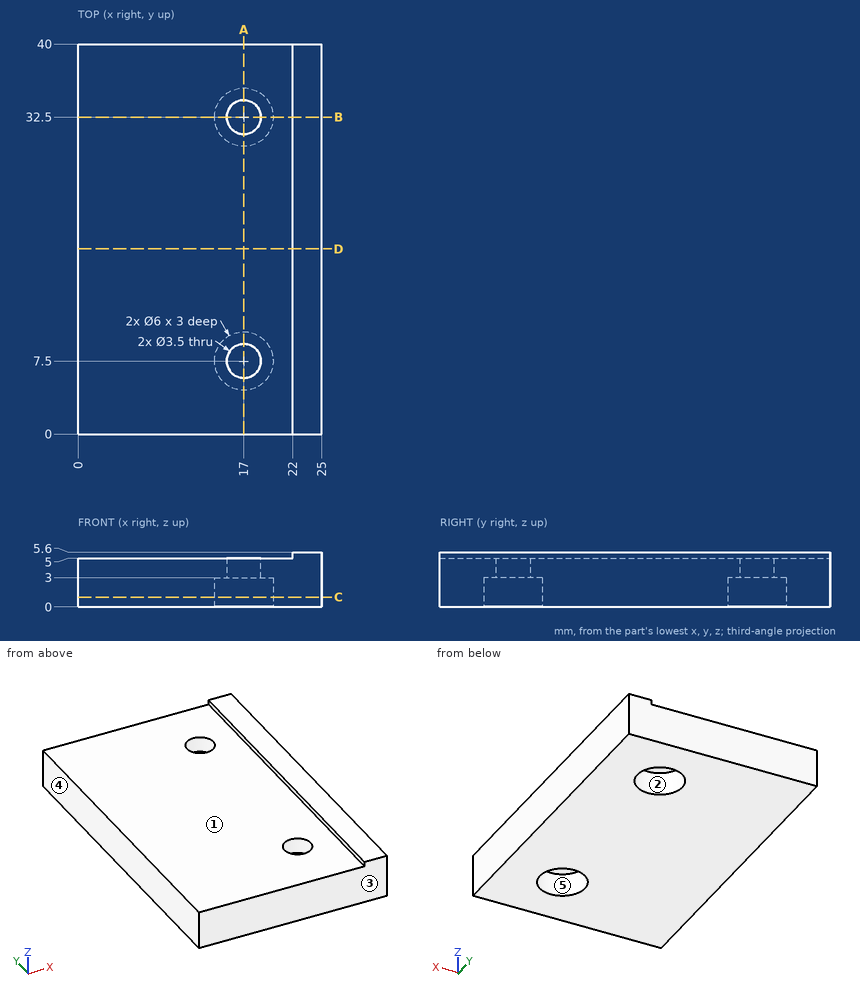
The drawing under review shows one solid part. Ordinate dimensions are in mm from its lowest x, y, z. A direction names the side the tool comes from. Round coordinates to 2 decimals unless told otherwise and drop trailing zeros. Order: outer loops, then holes, each group sorted by start corner. A loop starts at its lowest first (then second) coordinate and runs counter-clockwise, first axis right, second up. Notation, with made-up numbers: (6.25, 3.5) -> (45.25, 3.5) arc R28 cw to (45.25, 32.5) -> close; hole circle Ø3 at (-25.5, -10.5). An arc over 180 degrees is marked (long way). Return JSON: item names as keys, results as strings.
1. The part is to be moulded in two halves that separate along Y. For the marked faces 1, 2 and 3, say which applies: +Y half, -Y half, draft (parallel to the pull), parting line (faces both ways), or undercut.
Answer block:
{"face 1": "draft", "face 2": "undercut", "face 3": "-Y half"}
2. For L1, parallel to Y at x = 17, z = 3.8; L2, parallel to Y at x = 17, z = 0.7; L3, parallel to Z at x = 6.25, y = 6, list the stretches that pass through material, from the lowest coordinate up. Write a range as [from, to].
Answer block:
{"L1": "y = [0, 5.75], [9.25, 30.75], [34.25, 40]", "L2": "y = [0, 4.5], [10.5, 29.5], [35.5, 40]", "L3": "z = [0, 5]"}
3. Take a section at A-A (x = 17). Write out the cut boundary in (y, z), then the cut area to 3 significant figures.
Answer block:
{"outline": "(0, 0) -> (4.5, 0) -> (4.5, 3) -> (5.75, 3) -> (5.75, 5) -> (0, 5) -> close; (9.25, 3) -> (10.5, 3) -> (10.5, 0) -> (29.5, 0) -> (29.5, 3) -> (30.75, 3) -> (30.75, 5) -> (9.25, 5) -> close; (34.25, 3) -> (35.5, 3) -> (35.5, 0) -> (40, 0) -> (40, 5) -> (34.25, 5) -> close", "area": "150 mm²"}
4. Take a section at B-B (y = 32.5). Write out the cut boundary in (x, z).
Answer block:
{"outline": "(0, 0) -> (14, 0) -> (14, 3) -> (15.25, 3) -> (15.25, 5) -> (0, 5) -> close; (18.75, 3) -> (20, 3) -> (20, 0) -> (25, 0) -> (25, 5.6) -> (22, 5.6) -> (22, 5) -> (18.75, 5) -> close"}
5. Take a section at C-C (z = 1). Write out the cut boundary in (x, y), then the cut area to 3 significant figures.
Answer block:
{"outline": "(0, 0) -> (25, 0) -> (25, 40) -> (0, 40) -> close; hole circle Ø6 at (17, 7.5); hole circle Ø6 at (17, 32.5)", "area": "943 mm²"}
6. Insertion check: P1, Ø6.5, axis at x = 8, y = 18.5, coming from the +Z side; P2, Ø3, axis at x = 17, y = 8.5, coming from the -Z side. Each pin has a flat end and moves straight along its axis. Give the tip position at first contact, or say it passes through.
Answer block:
{"P1": "stops at z = 5", "P2": "stops at z = 3"}
7. For the marked faces 4 and 5, list the 3-axis set-ups (+Z, -Z, +X, -X, +Y, -Y) from which the entire face can be reached by the end or side of a thin tool; tool diameter is ignored.
Answer block:
{"face 4": "+Z, -Z, -X, +Y, -Y", "face 5": "-Z"}
8. Take a section at D-D (y = 19). Write out the cut boundary in (x, z), then the cut area to 3 significant figures.
Answer block:
{"outline": "(0, 0) -> (25, 0) -> (25, 5.6) -> (22, 5.6) -> (22, 5) -> (0, 5) -> close", "area": "127 mm²"}
